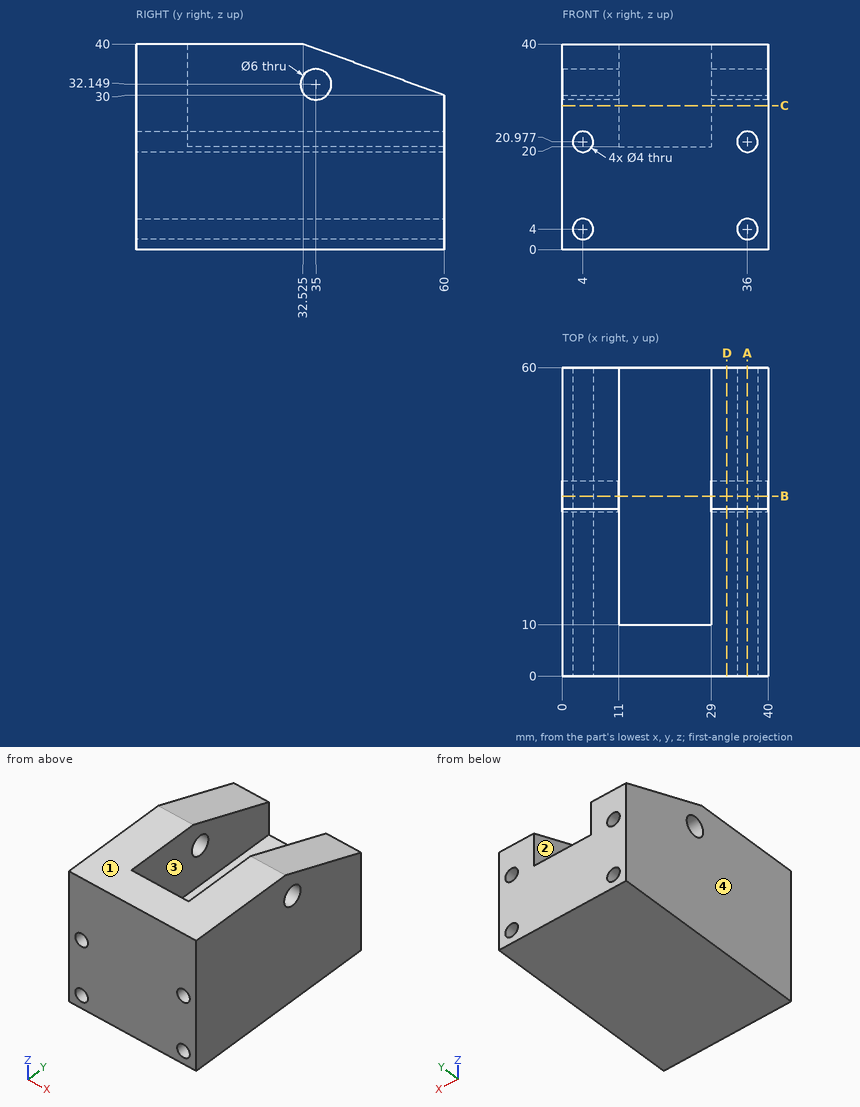
Job drawing, mm, ordinate dimensions from the low corner. One solid piece. Give positions to 0.01 mm unless a question says otherwise; leave off trailing zeros. Write each loop counter-clockwise with the first axis right and the second up, starting at its lowest first coordinate (ties: lowest second). Pieces come first, ordered by that corner, then holes. Notation, with made-up numbers: M 74.25,69.25 L 123.25,69.25 A16 cw 123.25,99.25 Z; hole C 89,25 d10. An arc over 180 degrees is marked long. Put each result on its own line as item: value. Start each with the question number.
(1) Band-saw the part on B-B, the plane y = 35. Write the cut outline in (x, z).
(2) Flat gauge pins, fed straight in: pin 1 Ø8 at (y, z) = (35, 32.15) entering from +X; pin 2 Ø14.5 at (x, z) = (20, 28.5) entering from +Y; pin 3 Ø9 at (x, y) = (21.5, 30) entering from +Z. Where does each tip first touch, or does it go through?
(3) Probe L1, parallel to X at y = 27, z = 4; L2, parallel to Z at x = 4, y = 27; L3, parallel to Z at x = 4, y = 36.5. List the from-to ranges inside material, lowest first.
(4) Band-saw the part on A-A, the plane x = 36. Write the cut outline in (y, z) (1 decimal), and give its area (3 significant figures).
(5) Mould opens along X. For the marked faces 1, 2, 3 and 4 say: +X half, -X half, draft (parallel to the pull), parting line (faces both ways), or undercut.
(6) Band-saw the part on C-C, the plane z = 28. Write the cut outline in (x, y).
(7) Band-saw the part on D-D, the plane x = 32. Write the cut outline in (y, z) (1 decimal).
Response values:
1. outline: M 0,0 L 40,0 L 40,29.15 L 29,29.15 L 29,20 L 11,20 L 11,29.15 L 0,29.15 Z; M 0,35.15 L 11,35.15 L 11,39.1 L 0,39.1 Z; M 29,35.15 L 40,35.15 L 40,39.1 L 29,39.1 Z; hole C 4,4 d4; hole C 4,20.98 d4; hole C 36,4 d4; hole C 36,20.98 d4
2. pin 1: stops at x = 40
2. pin 2: stops at y = 10
2. pin 3: stops at z = 20
3. L1: x = 0 to 2, 6 to 34, 38 to 40
3. L2: z = 0 to 2, 6 to 18.98, 22.98 to 40
3. L3: z = 0 to 2, 6 to 18.98, 22.98 to 29.55, 34.75 to 38.55
4. outline: M 0,0 L 60,0 L 60,2 L 0,2 Z; M 0,6 L 60,6 L 60,19 L 0,19 Z; M 0,23 L 60,23 L 60,30 L 32.5,40 L 0,40 Z; hole C 35,32.1 d6
4. area: 1,750 mm2
5. face 1: draft
5. face 2: undercut
5. face 3: undercut
5. face 4: -X half
6. outline: M 0,0 L 40,0 L 40,60 L 29,60 L 29,10 L 11,10 L 11,60 L 0,60 Z
7. outline: M 0,0 L 60,0 L 60,30 L 32.5,40 L 0,40 Z; hole C 35,32.1 d6
